For this review, take the finished solid that the model builds, in its own axes (mm). A direction names the side the tool comes from. Round coordinates to 2 decimals unless told otherwise and drop trailing zeros. Order: outer loops, then holes, each group sorted by start corner. A loop starts at its lowest first (then second) coordinate and runs counter-clockwise, first axis right, second up.
Autodesk Fusion 360 part; units mm, degrees
sketch "Sketch1" plane through (0, 0, 0) normal (0, 0, 1) x (1, 0, 0)
  circle A0 centre (0, 0) radius 10
  circle A1 centre (0, 0) radius 7.5 construction
  circle A2 centre (0, 7.5) radius 1.5
  circle A3 centre (-7.5, 0) radius 1.5
  circle A4 centre (0, -7.5) radius 1.5
  circle A5 centre (7.5, 0) radius 1.5
  line L0 (0, 7.5) -> (0, 0) construction
  circle A6 centre (0, 0) radius 4.5
  circle A7 centre (0, 0) radius 1.6
  circle A8 centre (0, 0) radius 3
  dimension "d1" = 20
  dimension "d2" = 15
  dimension "d3" = 3
  dimension "d6" = 360
  dimension "d7" = 9
  dimension "d8" = 3.2
  dimension "d9" = 6
extrude "Extrude1" add sketch "Sketch1" against normal blind 2.5 contours A0 | A6 | A8
extrude "Extrude2" add sketch "Sketch1" along normal blind 1.5 contours A6
fillet "Fillet1" radius 0.5 1 edges at (-4.1955, 1.6273, 0)
move_face "OffsetFaces1" offset -2 1 faces at (2.5162, -0.2285, 0)
thread "Thread1" thread offset 0 thread length 10
Q1. Mouldability with a two-part tool opening along Y and no side actions: class faces 3 (the face through (-2.17, -9.76, -1.23)), 4 (the face through (1.3, -1.3, -2)), 5 (the face through (2, 0, -2.5)) as +Y half, -Y half, draft (parallel to the pull), parting line (faces both ways), or undercut.
Q2. Wall thickness on line 1 (Y direction, x = 0, z = -1.1); line 2 (Y direction, x = 0, z = -2.15); line 3 (Z direction, x = 1, y = 5): over which ranges is each line inside the solid? List them lowest first.
Q3. Tool access review of faces 1 (the face through (0, -9, -1)), 2 (the face through (2, 5, 0)): name each direction out of +Z, -Z, +X, -X, +Y, -Y from which nothing blocks a thin tool from reaching the whole face with its end or side.
Q4. Take a section at D-D, the plane y = 6.75. State the section outline as (x, z) points, plus the area to 3 significant figures.
Q5. Take a section at A-A, the plane x = 0. State the section outline as (y, z) points, plus the area to 3 significant figures.
Q6. Clearance check with flat-ended pins moving along their axes: pin 1 (3 mm diameter, centred on x = 6, y = 6, fed in from +Z); pin 2 (2 mm diameter, centred on x = 8, z = -1.5, fed in from +Y). State where each tip first meets the part, or that it passes through.
Q7. Take a section at C-C, the plane x = -8.25. State the section outline as (y, z) points, plus the area to 3 significant figures.
Working result:
1. face 3: parting line
1. face 4: undercut
1. face 5: draft
2. line 1: y = -10 to -9, -6 to -3, 3 to 6, 9 to 10
2. line 2: y = -10 to -9, -6 to -1.6, 1.6 to 6, 9 to 10
2. line 3: z = -2.5 to 0
3. face 1: +Z, -Z
3. face 2: +Z
4. outline: (-7.38, -2.5) - (-1.3, -2.5) - (-1.3, 0) - (-7.38, 0) - close; (1.3, -2.5) - (7.38, -2.5) - (7.38, 0) - (1.3, 0) - close
4. area: 30.4 mm2
5. outline: (-10, -2.5) - (-9, -2.5) - (-9, 0) - (-10, 0) - close; (-6, -2.5) - (-1.6, -2.5) - (-1.6, -2) - (-3, -2) - (-3, 1.5) - (-4.5, 1.5) - (-4.5, 0.5) arc R0.5 cw to (-5, 0) - (-6, 0) - close; (1.6, -2.5) - (6, -2.5) - (6, 0) - (5, 0) arc R0.5 cw to (4.5, 0.5) - (4.5, 1.5) - (3, 1.5) - (3, -2) - (1.6, -2) - close; (9, -2.5) - (10, -2.5) - (10, 0) - (9, 0) - close
5. area: 26.0 mm2
6. pin 1: stops at z = 0
6. pin 2: stops at y = 7.14
7. outline: (-5.65, -2.5) - (-1.3, -2.5) - (-1.3, 0) - (-5.65, 0) - close; (1.3, -2.5) - (5.65, -2.5) - (5.65, 0) - (1.3, 0) - close
7. area: 21.8 mm2
